Input: part model. Units: mm. Frame: model coordinates. Face numbers are marked on the shaded views. Coordinates: 2 decimals unless noted, no trailing zeros. Order: outer loops, then holes, each group sorted by start corner. A loop starts at its lowest first (then second) coordinate and runs counter-clockwise, first axis right, second up. Notation, with made-up numbers: M 34,65.25 L 49,65.25 A29 ccw 49,97.25 Z; hole C 56.25,82 d2. An arc over 180 degrees is marked long. One line per item, written item: value.
```python
from build123d import *

# Parameters (mm, degrees)
SKETCH1_R           = 9
SKETCH1_R_2         = 1.5
BOSS_EXTRUDE1_DEPTH = 1
SKETCH2_R           = 6
SKETCH2_R_2         = 1.5
BOSS_EXTRUDE2_DEPTH = 11
SKETCH3_R           = 9
SKETCH3_R_2         = 1.5
BOSS_EXTRUDE3_DEPTH = 1


with BuildPart() as part:
    # Sketch1 → Boss-Extrude1 (new body)
    with BuildSketch(Plane(origin=(0, 0, 0), x_dir=(0, 0, -1), z_dir=(1, 0, 0))):
        Circle(SKETCH1_R)
        Circle(SKETCH1_R_2, mode=Mode.SUBTRACT)
    extrude(amount=BOSS_EXTRUDE1_DEPTH)

    # Sketch2 → Boss-Extrude2 (add)
    with BuildSketch(Plane(origin=(1, 0, 0), x_dir=(0, 0, -1), z_dir=(1, 0, 0))):
        Circle(SKETCH2_R)
        Circle(SKETCH2_R_2, mode=Mode.SUBTRACT)
    extrude(amount=BOSS_EXTRUDE2_DEPTH)

    # Sketch3 → Boss-Extrude3 (add)
    with BuildSketch(Plane(origin=(12, 0, 0), x_dir=(0, 0, -1), z_dir=(1, 0, 0))):
        Circle(SKETCH3_R)
        Circle(SKETCH3_R_2, mode=Mode.SUBTRACT)
    extrude(amount=BOSS_EXTRUDE3_DEPTH)


solid = part.part
```
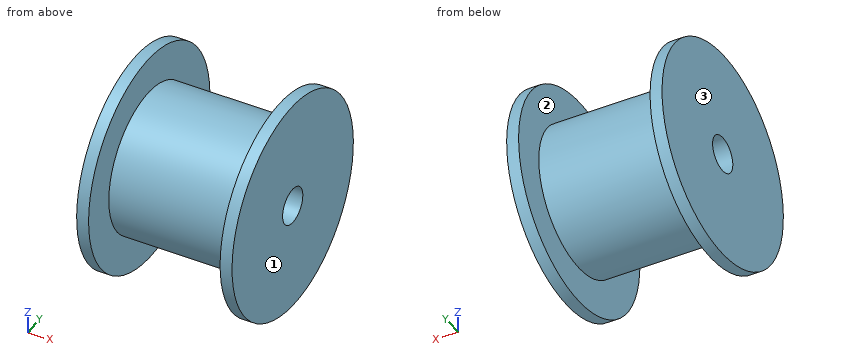
(1) Cut plane C-C on z = 4.5. Output: boundary loops of the cut face in (x, y), plus the area to 3 significant figures.
Data:
outline: M 0,-7.79 L 1,-7.79 L 1,-3.97 L 12,-3.97 L 12,-7.79 L 13,-7.79 L 13,7.79 L 12,7.79 L 12,3.97 L 1,3.97 L 1,7.79 L 0,7.79 Z
area: 118 mm2
(2) Ray query, line 1 (Y direction, x = 7.75, z = 0); line 2 (X direction, y = -6, z = -2.75); line 3 (Y direction, x = 6.75, z = -1). Return the intervals inside material, ascending. Write a range as from..to.
Data:
line 1: y = -6..-1.5, 1.5..6
line 2: x = 0..1, 12..13
line 3: y = -5.92..-1.12, 1.12..5.92
(3) First-contact query: pin 1 (4 mm diameter, centred on x = 9, z = -1, fed in from -Y); pin 2 (6 mm diameter, centred on x = 3.5, z = -4.5, fed in from +Y); pin 3 (2.5 mm diameter, centred on y = 0, z = 0, fed in from +X); pin 4 (1.5 mm diameter, centred on x = 2.5, y = 4, fed in from -Z). Flat tips, straight axial feed; report the tip coordinate or a pass-through.
Data:
pin 1: stops at y = -6
pin 2: stops at y = 8.54
pin 3: passes through
pin 4: stops at z = -5.04
(4) Cut plane D-D on y = -5.75. Output: boundary loops of the cut face in (x, z).
Data:
outline: M 0,-6.92 L 1,-6.92 L 1,-1.71 L 12,-1.71 L 12,-6.92 L 13,-6.92 L 13,6.92 L 12,6.92 L 12,1.71 L 1,1.71 L 1,6.92 L 0,6.92 Z
(5) Cut plane A-A on y = 0. Output: boundary loops of the cut face in (x, z).
Data:
outline: M 0,-9 L 1,-9 L 1,-6 L 12,-6 L 12,-9 L 13,-9 L 13,-1.5 L 0,-1.5 Z; M 0,1.5 L 13,1.5 L 13,9 L 12,9 L 12,6 L 1,6 L 1,9 L 0,9 Z
(6) Draft query along X for the marked faces 1, 2 and 3. Return one class per face: released by +X, released by -X, zero draft, split by the parting line, or undercut.
Data:
face 1: released by +X
face 2: undercut
face 3: released by -X
